Check sheet for the modelled part. Datum: model origin and axes. Units: mm. Face numbers are marked on the shaded views. A direction names the side the tool comes from. Round coordinates to 2 decimals unless told otherwise and drop trailing zeros. Write each loop counter-clockwise with the first axis right and the second up, starting at its lowest first coordinate (ties: lowest second). Pieces come first, ordered by that corner, then holes. Notation, with made-up numbers: (29.25, -35.75) -> (53.25, -35.75) arc R24 cw to (53.25, -0.75) -> close; hole circle Ø5 at (84.5, 40). An arc over 180 degrees is marked (long way). Write item = value, one per line.
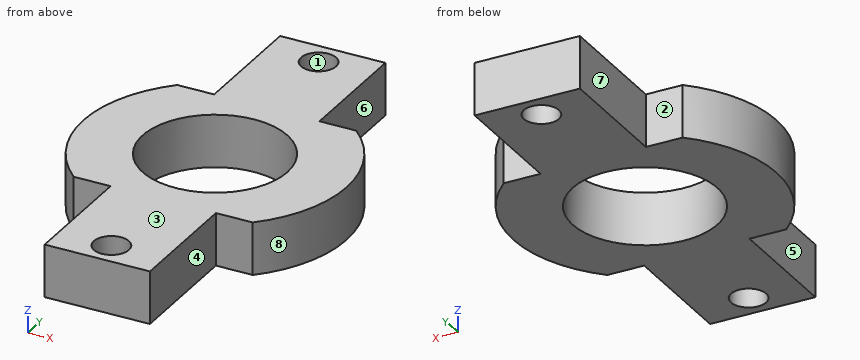
from build123d import *

# Parameters (mm, degrees)
SKETCH1_R           = 8.25
BOSS_EXTRUDE1_DEPTH = 6
SKETCH3_R           = 2
CUT_EXTRUDE1_DEPTH  = 30.765752132


with BuildPart() as part:
    # Sketch1 → Boss-Extrude1 (new body)
    with BuildSketch(Plane.XY):
        with BuildLine():
            Line((6, -25), (6, -11))
            Line((6, -11), (10.198039027, -11))
            ThreePointArc((10.198039027, -11), (15, 0), (10.198039027, 11))
            Line((10.198039027, 11), (6, 11))
            Line((6, 11), (6, 25))
            Line((6, 25), (-6, 25))
            Line((-6, 25), (-6, 11))
            Line((-6, 11), (-10.198039027, 11))
            ThreePointArc((-10.198039027, 11), (-15, 0), (-10.198039027, -11))
            Line((-10.198039027, -11), (-6, -11))
            Line((-6, -11), (-6, -25))
            Line((-6, -25), (6, -25))
        make_face()
        Circle(SKETCH1_R, mode=Mode.SUBTRACT)
    extrude(amount=BOSS_EXTRUDE1_DEPTH)

    # Sketch3 → Cut-Extrude1 (cut, through all)
    with BuildSketch(Plane(origin=(0, 0, 0), x_dir=(-1, 0, 0), z_dir=(0, 0, -1))):
        with Locations((0, 22)):
            Circle(SKETCH3_R)
        with Locations((0, -22)):
            Circle(SKETCH3_R)
    extrude(amount=-CUT_EXTRUDE1_DEPTH, mode=Mode.SUBTRACT)


solid = part.part
(1) Access from +Z, -Z, +X, -X, +Y, -Y to the whole of each face (thin tool, end or side, straight path). Record for the marked faces 4, 5, 6, 7 and 8.
Worked answers:
face_4 = +Z, -Z, +X, -Y
face_5 = +Z, -Z, -X, -Y
face_6 = +Z, -Z, +X, +Y
face_7 = +Z, -Z, -X, +Y
face_8 = +Z, -Z, +X
(2) Go/stop test with flat-tipped pins: P1, Ø3, axis at y = 15.5, z = 2, coming from the -X side; P2, Ø1.8, axis at y = 18.5, z = 2, coming from the +X side; P3, Ø5, axis at x = -2, y = -7.5, coming from the +Z side. Record where each tip stops, or that it passes through.
Worked answers:
P1 = -6
P2 = 6
P3 = 6
(3) Sectioned sample at B-B on x = 0. Enter the section's corners in (y, z), then the cut area to 3 significant figures.
Worked answers:
outline = (-25, 0) -> (-24, 0) -> (-24, 6) -> (-25, 6) -> close; (-20, 0) -> (-8.25, 0) -> (-8.25, 6) -> (-20, 6) -> close; (8.25, 0) -> (20, 0) -> (20, 6) -> (8.25, 6) -> close; (24, 0) -> (25, 0) -> (25, 6) -> (24, 6) -> close
area = 153 mm²
(4) Material ranges on L1, parallel to Y at x = 0, z = 4.15; L2, parallel to X at y = 14, z = 5.15; L3, parallel to Y at x = -3.75, z = 3.9, recorded low to high. Write a range as [from, to].
Worked answers:
L1 = [-25, -24], [-20, -8.25], [8.25, 20], [24, 25]
L2 = [-6, 6]
L3 = [-25, -7.35], [7.35, 25]
(5) Sectioned sample at C-C on z = 2.15. Enter the section's corners in (x, y), then the cut area to 3 significant figures.
Worked answers:
outline = (-10.2, -11) -> (-6, -11) -> (-6, -25) -> (6, -25) -> (6, -11) -> (10.2, -11) arc R15 ccw to (10.2, 11) -> (6, 11) -> (6, 25) -> (-6, 25) -> (-6, 11) -> (-10.2, 11) arc R15 ccw to start; hole circle Ø16.5 at (0, 0); hole circle Ø4 at (0, -22); hole circle Ø4 at (0, 22)
area = 692 mm²
(6) Release check for a two-part mould opening along Y. For the marked faces 1, 2 and 3 record: pulls with the +Y half, pulls with the -Y half, needs draft (parallel to the pull), parting line crosses it, or undercut.
Worked answers:
face_1 = undercut
face_2 = pulls with the +Y half
face_3 = needs draft
(7) Sectioned sample at A-A on y = -22. Enter the section's corners in (x, z).
Worked answers:
outline = (-6, 0) -> (-2, 0) -> (-2, 6) -> (-6, 6) -> close; (2, 0) -> (6, 0) -> (6, 6) -> (2, 6) -> close
(8) Sectioned sample at D-D on x = -6.75. Enter the section's corners in (y, z), then the cut area to 3 significant figures.
Worked answers:
outline = (-11, 0) -> (-4.74, 0) -> (-4.74, 6) -> (-11, 6) -> close; (4.74, 0) -> (11, 0) -> (11, 6) -> (4.74, 6) -> close
area = 75.1 mm²
